Could you check a few things on this drawing? It's one solid part, dimensions in mm from its lowest x, y, z. Give positions to 0.01 mm unless a question says otherwise; leave off trailing zeros. Write each loop counter-clockwise with the first axis right and the second up, starting at its lowest first coordinate (ties: lowest second). Pieces come first, ordered by that corner, then holes.
1. I'm going to push flat-ended pins straight in: pin 1 (6.5 mm diameter, centred on x = 65, y = 15, fed in from -Z); pin 2 (3 mm diameter, centred on x = 60.5, z = 5, fed in from -Y). Where does each tip first touch, or does it pass through?
2. Suppose I cut it at C-C (y = 15). Please give me the cut outline in (x, z).
3. Suppose I cut it at B-B (x = 65). Please give me the cut outline in (y, z).
4. If I drill on probe 1 along Y at (x, z) = (102.5, 5); probe 2 along Y at (x, z) = (14, 7.25); probe 3 along Z at (x, y) = (12.5, 17.25), over which ranges is the centre line in solid material (lowest first)?
5. Suppose I cut it at A-A (z = 5). Please give me the cut outline in (x, y), and give its area (3 significant figures).
6. Suppose I cut it at D-D (x = 12). Please give me the cut outline in (y, z), and give its area (3 significant figures).
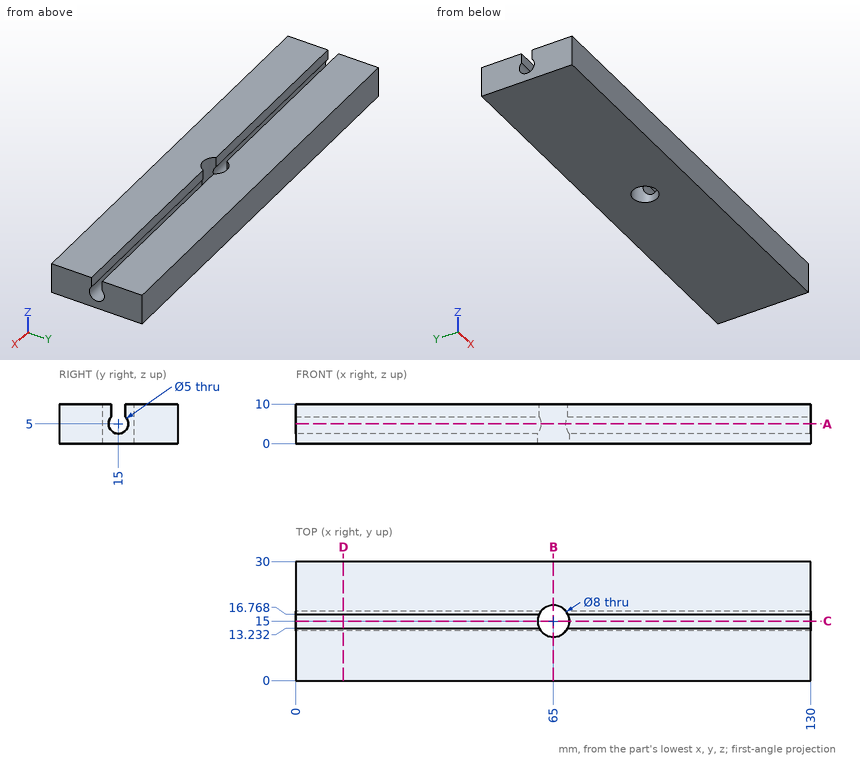
Checks:
1. pin 1: passes through
1. pin 2: stops at y = 0
2. outline: (0, 0) - (61, 0) - (61, 2.5) - (0, 2.5) - close; (69, 0) - (130, 0) - (130, 2.5) - (69, 2.5) - close
3. outline: (0, 0) - (11, 0) - (11, 10) - (0, 10) - close; (19, 0) - (30, 0) - (30, 10) - (19, 10) - close
4. probe 1: y = 0 to 12.5, 17.5 to 30
4. probe 2: y = 0 to 13.23, 16.77 to 30
4. probe 3: z = 0 to 3.91, 6.09 to 10
5. outline: (0, 0) - (130, 0) - (130, 12.5) - (68.12, 12.5) arc R4 cw to (61.88, 12.5) - (0, 12.5) - close; (0, 17.5) - (61.88, 17.5) arc R4 cw to (68.12, 17.5) - (130, 17.5) - (130, 30) - (0, 30) - close
5. area: 3,240 mm2
6. outline: (0, 0) - (30, 0) - (30, 10) - (16.77, 10) - (16.77, 6.77) arc R2.5 cw (long way) to (13.23, 6.77) - (13.23, 10) - (0, 10) - close
6. area: 271 mm2
